For this review, take the finished solid that the model builds, in its own axes (mm). Face numbers are marked on the shaded views. A direction names the side the tool comes from. Round coordinates to 2 decimals unless told otherwise and drop trailing zeros. Write each loop counter-clockwise with the first axis right and the second up, starting at its lowest first coordinate (ties: lowest second). Pieces come first, ordered by that corner, then holes. Notation, with made-up numbers: (-23.5, 37) - (0.5, 37) arc R16 cw to (0.5, 41) - close; hole circle Ø6 at (-39.5, 42.25). An arc over 180 degrees is marked (long way). Answer in a Markdown table with one row per item. Add a question column.
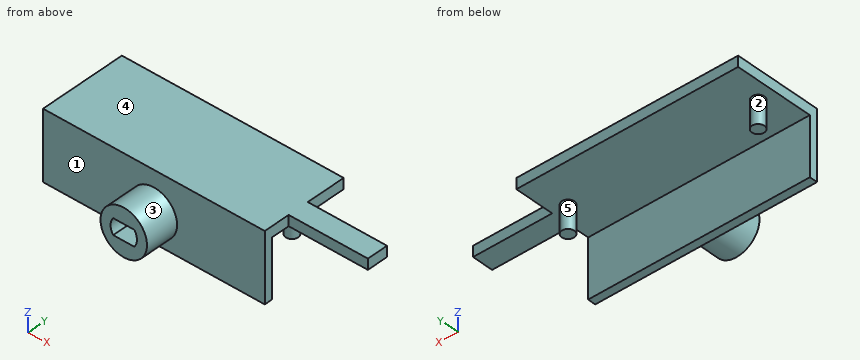
from build123d import *

# Parameters (mm, degrees)
ESQUISSE1_W        = 42
ESQUISSE1_H        = 15
BOSS_EXTRU_1_DEPTH = 2
ESQUISSE2_R        = 1.175
BOSS_EXTRU_2_DEPTH = 5.2
ESQUISSE3_W        = 2
ESQUISSE3_H        = 4
BOSS_EXTRU_3_DEPTH = 15
ESQUISSE4_W        = 42
ESQUISSE4_H        = 2
BOSS_EXTRU_4_DEPTH = 1.5
ESQUISSE5_W        = 42
ESQUISSE5_H        = 1.5
BOSS_EXTRU_5_DEPTH = 11
ESQUISSE6_R        = 4.402379767
BOSS_EXTRU_6_DEPTH = 6.3


with BuildPart() as part:
    # Esquisse1 → Boss.-Extru.1 (new body)
    with BuildSketch(Plane.XY):
        with Locations((21, 7.5)):
            Rectangle(ESQUISSE1_W, ESQUISSE1_H)
    extrude(amount=BOSS_EXTRU_1_DEPTH)

    # Esquisse2 → Boss.-Extru.2 (add)
    with BuildSketch(Plane(origin=(0, 0, 0), x_dir=(-1, 0, 0), z_dir=(0, 0, -1))):
        with Locations((-39, 7.5)):
            Circle(ESQUISSE2_R)
        with Locations(Location((-3, 7.5, 0), (0, 0, 180))):
            Circle(ESQUISSE2_R)
    extrude(amount=BOSS_EXTRU_2_DEPTH)

    # Esquisse3 → Boss.-Extru.3 (add)
    with BuildSketch(Plane(origin=(42, 0, 0), x_dir=(0, 0, -1), z_dir=(1, 0, 0))):
        with Locations((-1, 5.5)):
            Rectangle(ESQUISSE3_W, ESQUISSE3_H)
    extrude(amount=BOSS_EXTRU_3_DEPTH)

    # Esquisse4 → Boss.-Extru.4 (add)
    with BuildSketch(Plane.XZ):
        with Locations((21, 1)):
            Rectangle(ESQUISSE4_W, ESQUISSE4_H)
    extrude(amount=BOSS_EXTRU_4_DEPTH)

    # Esquisse5 → Boss.-Extru.5 (add)
    with BuildSketch(Plane(origin=(0, 0, 0), x_dir=(-1, 0, 0), z_dir=(0, 0, -1))):
        with Locations((-21, -0.75)):
            Rectangle(ESQUISSE5_W, ESQUISSE5_H)
    extrude(amount=BOSS_EXTRU_5_DEPTH)

    # Esquisse6 → Boss.-Extru.6 (add)
    with BuildSketch(Plane.XZ.offset(1.5)):
        with Locations(Location((21, -5.5, 0), (0, 0, 270))):
            Circle(ESQUISSE6_R)
        with BuildLine():
            Line((19.002059064, -7.0027415), (22.997940936, -7.0027415))
            ThreePointArc((22.997940936, -7.0027415), (23.499997651, -5.503426877), (23.002053192, -4.0027415))
            Line((23.002053192, -4.0027415), (18.997946808, -4.0027415))
            ThreePointArc((18.997946808, -4.0027415), (18.500002349, -5.503426877), (19.002059064, -7.0027415))
        make_face(mode=Mode.SUBTRACT)
    extrude(amount=BOSS_EXTRU_6_DEPTH)


solid = part.part
Q1. Add section D-D on x = 35. State the section outline as (y, z) points.
Q2. Add section C-C on x = 3. State the section outline as (y, z) points (3 decimals), then the cut area to 3 significant figures.
Q3. To check wall thickness, follow probe 1 along Z at (x, y) = (17, 8.75); probe 2 along Y at (x, z) = (54, 1.5); probe 3 along Y at (x, z) = (4, -0.5). State the ranges of each line that lie inside material, in increasing order.
Q4. Insertion check: pin 1 Ø1 at (x, y) = (22, 3.5) entering from -Z; pin 2 Ø5.5 at (y, z) = (1, -3.5) entering from +X; pin 3 Ø0.7 at (x, y) = (39.5, 7) entering from -Z. Each pin has a flat end and moves straight along its axis. Give the tip position at first contact, or say it passes through.
Q5. Add section B-B on z = -6. State the section outline as (x, y) points.
Q6. Tool access review of the marked faces 4 and 5: name each direction out of +Z, -Z, +X, -X, +Y, -Y from which nothing blocks a thin tool from reaching the whole face with its end or side.
Q7. Draft analysis for pull direction Y (two halves, no side actions). For the marked faces 1, 2 and 3, state which applies: released by +Y, released by -Y, zero draft, split by the parting line, or undercut.
Q8. Add section A-A on x = 21. State the section outline as (y, z) points, then the cut area to 3 significant figures.
Answer sheet:
| question | item | result |
|---|---|---|
| 1 | outline | (-1.5, -11) - (0, -11) - (0, 0) - (15, 0) - (15, 2) - (-1.5, 2) - close |
| 2 | outline | (-1.5, -11) - (0, -11) - (0, 0) - (6.325, 0) - (6.325, -5.2) - (8.675, -5.2) - (8.675, 0) - (15, 0) - (15, 2) - (-1.5, 2) - close |
| 2 | area | 61.7 mm² |
| 3 | probe 1 | z = 0 to 2 |
| 3 | probe 2 | y = 3.5 to 7.5 |
| 3 | probe 3 | y = -1.5 to 0, 6.88 to 8.12 |
| 4 | pin 1 | stops at z = 0 |
| 4 | pin 2 | stops at x = 42 |
| 4 | pin 3 | stops at z = -5.2 |
| 5 | outline | (0, -1.5) - (16.63, -1.5) - (16.63, -7.8) - (18.55, -7.8) - (18.55, -1.5) - (23.45, -1.5) - (23.45, -7.8) - (25.37, -7.8) - (25.37, -1.5) - (42, -1.5) - (42, 0) - (0, 0) - close |
| 6 | face 4 | +Z, +X, -X, +Y, -Y |
| 6 | face 5 | -Z |
| 7 | face 1 | released by -Y |
| 7 | face 2 | undercut |
| 7 | face 3 | zero draft |
| 8 | outline | (-7.8, -9.9) - (-1.5, -9.9) - (-1.5, -11) - (0, -11) - (0, 0) - (15, 0) - (15, 2) - (-1.5, 2) - (-1.5, -1.1) - (-7.8, -1.1) - (-7.8, -4) - (-1.5, -4) - (-1.5, -7) - (-7.8, -7) - close |
| 8 | area | 86.1 mm² |
